from build123d import *

# Parameters (mm, degrees)
SKETCH1_R           = 1.5
SKETCH1_R_2         = 2
SKETCH1_R_3         = 7
BOSS_EXTRUDE1_DEPTH = 10


with BuildPart() as part:
    # Sketch1 → Boss-Extrude1 (new body)
    with BuildSketch(Plane(origin=(0, 0, 0), x_dir=(1, 0, 0), z_dir=(0, 1, 0))):
        with BuildLine():
            ThreePointArc((53.57700678, 17.304163694), (50.585779575, 15.593662693), (47.191546456, 15))
            Line((47.191546456, 15), (0, 15))
            Line((0, 15), (0, 0))
            Line((0, 0), (47.191546456, 0))
            ThreePointArc((47.191546456, 0), (50.585779575, -0.593662693), (53.57700678, -2.304163694))
            Line((53.57700678, -2.304163694), (56.126078821, -4.419203273))
            ThreePointArc((56.126078821, -4.419203273), (82.8, 7.5), (56.126078821, 19.419203273))
            Line((56.126078821, 19.419203273), (53.57700678, 17.304163694))
        make_face()
        with Locations(Location((12.7, 7.5, 0), (0, 0, 270))):
            Circle(SKETCH1_R, mode=Mode.SUBTRACT)
        with Locations(Location((25.4, 7.5, 0), (0, 0, 270))):
            Circle(SKETCH1_R, mode=Mode.SUBTRACT)
        with Locations(Location((38.1, 7.5, 0), (0, 0, 270))):
            Circle(SKETCH1_R, mode=Mode.SUBTRACT)
        with BuildLine():
            ThreePointArc((53.4862915, 7.5), (55.4862915, 9.5), (57.4862915, 7.5))
            ThreePointArc((57.4862915, 7.5), (55.4862915, 5.5), (53.4862915, 7.5))
        make_face(mode=Mode.SUBTRACT)
        with Locations(Location((66.8, -3.8137085, 0), (0, 0, 270))):
            Circle(SKETCH1_R_2, mode=Mode.SUBTRACT)
        with Locations(Location((66.8, 18.8137085, 0), (0, 0, 270))):
            Circle(SKETCH1_R_2, mode=Mode.SUBTRACT)
        with Locations(Location((78.1137085, 7.5, 0), (0, 0, 270))):
            Circle(SKETCH1_R_2, mode=Mode.SUBTRACT)
        with Locations(Location((66.8, 7.5, 0), (0, 0, 270))):
            Circle(SKETCH1_R_3, mode=Mode.SUBTRACT)
    extrude(amount=BOSS_EXTRUDE1_DEPTH)


solid = part.part
The listing builds one solid part. Answer for the finished solid, in the listing's coordinates (mm). A direction names the side the tool comes from. Round coordinates to 2 decimals unless told otherwise and drop trailing zeros. Write each loop counter-clockwise with the first axis right and the second up, starting at its lowest first coordinate (ties: lowest second). Pieces come first, ordered by that corner, then holes. Notation, with made-up numbers: (-35.5, -21) - (23.5, -21) arc R18 cw to (23.5, -11) - close; hole circle Ø8 at (24.25, -12.75). An arc over 180 degrees is marked (long way). Use a Markdown table: item, result. Add a question column.
1. A tool of negligible diameter and unlimited length cuts with its end or side. For faces 4 (the face through (23, 5, 0)), 5 (the face through (41, 0, -8)), 6 (the face through (24, 5, -15)), from which of +Z, -Z, +X, -X, +Y, -Y can it reach the whole face along a straight path? Write none if from no direction.
2. Consider line 1 (Z direction, x = 67, y = 3.5); line 2 (Z direction, x = 15, y = 3); line 3 (Z direction, x = 70, y = 3). Determine where each line is inside the solid, lowest interval first.
3. For a pull along Z with two mould halves and no side action, classify faces 1 (the face through (41, 10, -8)), 2 (the face through (82.79, 4.93, -6.98)), 3 (the face through (80.097, 4.93, -7.76)) as +Z half, -Z half, draft (parallel to the pull), parting line (faces both ways), or undercut.
4. Flat-ended cylindrical pins translate along their axes: P1, Ø11, axis at x = 66.8, z = -7.5, coming from the -Y side; P2, Ø1, axis at x = 10, y = 2.5, coming from the -Z side; P3, Ø3, axis at x = 29.5, y = 5, coming from the +Z side. Find the tip coordinate at first contact, or state that the pin passes through.
5. The part is cut by section D-D (x = 28). Write down the section's boundary in (y, z).
6. The part is cut by section A-A (x = 38.1). Write down the section's boundary in (y, z).
7. The part is cut by section B-B (y = 8). Give the number of separate pieces and of enclosed holes in the cut face, and give its area (3 significant figures).
8. The part is cut by section C-C (z = -2). Write down the section's boundary in (x, y), and give its area (3 significant figures).
Reported:
| question | item | result |
|---|---|---|
| 1 | face 4 | +Z, -X, +Y, -Y |
| 1 | face 5 | +Z, -Z, +X, -X, -Y |
| 1 | face 6 | -Z, -X, +Y, -Y |
| 2 | line 1 | -23.5 to -20.8, -16.82 to -14.5, -0.5 to 1.82, 5.8 to 8.5 |
| 2 | line 2 | -15 to 0 |
| 2 | line 3 | -23.18 to -13.73, -1.27 to 8.18 |
| 3 | face 1 | draft |
| 3 | face 2 | parting line |
| 3 | face 3 | undercut |
| 4 | P1 | through |
| 4 | P2 | z = -15 |
| 4 | P3 | z = 0 |
| 5 | outline | (0, -15) - (10, -15) - (10, 0) - (0, 0) - close |
| 6 | outline | (0, -15) - (10, -15) - (10, -9) - (0, -9) - close; (0, -6) - (10, -6) - (10, 0) - (0, 0) - close |
| 7 | separate pieces | 1 |
| 7 | enclosed holes | 8 |
| 7 | area | 1,360 mm^2 |
| 8 | outline | (0, 0) - (62.47, 0) - (62.47, 10) - (0, 10) - close; (71.13, 0) - (81.82, 0) - (81.82, 10) - (71.13, 10) - close |
| 8 | area | 732 mm^2 |
